Could you check a few things on this model? Use its own coordinates, in mm. Give positions to 0.01 mm unless a question says otherwise; leave off trailing zeros. Write each loop counter-clockwise with the first axis right and the second up, starting at its lowest first coordinate (ties: lowest second). Pieces come first, ordered by that corner, then holes. Notation, with made-up numbers: (20.5, 87) - (58.5, 87) arc R20 cw to (58.5, 112) - close; hole circle Ø2 at (84, -21). An arc over 180 degrees is marked (long way). Answer as a JSON object with one key per item and string values. Group by question number.
Autodesk Inventor part; units mm, degrees
ref_plane "YZ Plane" through (0, 0, 0) normal (1, 0, 0) x (0, 1, 0)
ref_plane "XZ Plane" through (0, 0, 0) normal (0, 1, 0) x (-1, 0, 0)
ref_plane "XY Plane" through (0, 0, 0) normal (0, 0, 1) x (1, 0, 0)
sketch "Sketch1" plane through (0, 0, 0) normal (0, 0, 1) x (1, 0, 0)
  arc A0 (-73.7988, 68.3559) -> (-25.1062, 68.3559) centre (-49.4525, 70.5784) ccw
  arc A1 (-70.366, 68.3559) -> (-28.5391, 68.3559) centre (-49.4525, 70.5784) ccw
  line L0 (-73.7988, 68.3559) -> (-70.366, 68.3559)
  line L1 (-28.5391, 68.3559) -> (-25.1062, 68.3559)
  dimension "d0" = 22.225
  dimension "d1" = 21.0312
  dimension "d2" = 24.4475
extrude "Extrusion1" add sketch "Sketch1" along normal blind 25.4
fillet "Fillet1" radius 9.525 2 edges at (-72.0824, 68.3559, 25.4) (-26.8227, 68.3559, 25.4)
properties part number "FE-00006-08"
(1) I want a section at A-A, the plane y = 51.5. Please give me the cut outline in (x, z), and give its area (3 significant figures).
(2) Will these pins go through, and if not, where does the flat tip stop? P1, Ø12, axis at x = -62.5, y = 60, coming from the -Z side; P2, Ø8, axis at x = -42, z = 22, coming from the -Y side; P3, Ø6, axis at x = -38.5, z = 4.5, coming from the -Y side; P4, Ø1, axis at x = -50, z = 5, coming from the +Y side.
(3) If we mould it in two halves opening along X, with no side actions, what happens to faces 1 (the flat face through (-27, 68.356, 8)), 2 (the cylindrical face through (-49.02, 49.55, 12.52)), 3 (the cylindrical face through (-48.946, 46.136, 12.522))? For each: +X half, -X half, draft (parallel to the pull), parting line (faces both ways), or undercut.
(4) I need wall thicknesses on L1, parallel to X at y = 59.5, z = 10.5; L2, parallel to X at y = 61.25, z = 21.75; L3, parallel to Z at x = -70, y = 59.25. Which ranges of each line are inside material? Lowest first, please.
(5) I want a section at C-C, the plane y = 63. Please give me the cut outline in (x, z), and give its area (3 significant figures).
Entries:
{
 "1": {"outline": "(-64.74, 0) - (-58.3, 0) - (-58.3, 25.4) - (-64.74, 25.4) - close; (-40.6, 0) - (-34.17, 0) - (-34.17, 25.4) - (-40.6, 25.4) - close", "area": "327 mm^2"},
 "2": {"P1": "z = 0", "P2": "y = 46.38", "P3": "y = 47.46", "P4": "y = 49.57"},
 "3": {"face 1": "draft", "face 2": "undercut", "face 3": "parting line"},
 "4": {"L1": "-71.25 to -67.33, -31.58 to -27.66", "L2": "-72.05 to -68.3, -30.6 to -26.85", "L3": "0 to 25.39"},
 "5": {"outline": "(-72.7, 0) - (-69.07, 0) - (-69.07, 24.44) - (-72.7, 24.44) - close; (-29.83, 0) - (-26.21, 0) - (-26.21, 24.44) - (-29.83, 24.44) - close", "area": "177 mm^2"}
}
